Source: CAD feature listing. Evaluate the final solid. Frame: model axes, mm. A direction names the side the tool comes from. Give positions to 0.01 mm unless a question says otherwise; leave off trailing zeros. Put each result on its own line as item: value.
```python
from build123d import *
from build123d.topology import SkipClean

# Parameters (mm, degrees)
BOSS_EXTRUDE1_DEPTH = 640
SKETCH22_R          = 6
CUT_EXTRUDE4_DEPTH  = 10
BOSS_EXTRUDE2_DEPTH = 63
BOSS_EXTRUDE3_DEPTH = 7
SKETCH26_R          = 6
CUT_EXTRUDE5_DEPTH  = 7
FILLET1_R           = 10
FILLET2_R           = 10
FILLET3_R           = 5
FILLET5_R           = 1


with BuildPart() as part:
    # Sketch1 → Boss-Extrude1 (new body)
    with BuildSketch(Plane.XY):
        Polygon((0, 0), (0, 70), (70, 70), (70, 63), (7, 63), (7, 0), align=None)
    extrude(amount=BOSS_EXTRUDE1_DEPTH)

    # Sketch22 → Cut-Extrude4 (cut)
    with BuildSketch(Plane(origin=(0, 70, 0), x_dir=(1, 0, 0), z_dir=(0, 1, 0))):
        with Locations((35, 0)):
            Circle(SKETCH22_R)
        with Locations((35, 500)):
            Circle(SKETCH22_R)
        with Locations(Location((35, -500, 0), (0, 0, 270))):
            Circle(SKETCH22_R)
    extrude(amount=-CUT_EXTRUDE4_DEPTH, mode=Mode.SUBTRACT)

    # Sketch23 → Boss-Extrude2 (add)
    with BuildSketch(Plane(origin=(0, 0, 0), x_dir=(1, 0, 0), z_dir=(0, 1, 0))):
        Polygon((0, -640), (42.5, -713.612159322), (48.562177826, -710.112159322), (7, -640), align=None)
    extrude(amount=BOSS_EXTRUDE2_DEPTH)

    # Sketch25 → Boss-Extrude3 (add)
    with BuildSketch(Plane(origin=(0, 63, 0), x_dir=(1, 0, 0), z_dir=(0, 1, 0))):
        Polygon((70, -640), (0, -640), (42.5, -713.612159322), (70, -713.612159322), align=None)
    extrude(amount=BOSS_EXTRUDE3_DEPTH)

    # Sketch26 → Cut-Extrude5 (cut)
    with BuildSketch(Plane(origin=(-275.556719825, 0, 163.348804279), x_dir=(-0.5099316128113042, 0, -0.8602149442178172), z_dir=(0.8602149442178172, 0, -0.5099316128113042))):
        with Locations((-614.36248118, 31.5)):
            Circle(SKETCH26_R)
        with Locations((-575.367085589, 31.5)):
            Circle(SKETCH26_R)
    extrude(amount=-CUT_EXTRUDE5_DEPTH, mode=Mode.SUBTRACT)

    # Mirror1: part across plane


with BuildPart() as part_1:
    with SkipClean():  # the faces are left unmerged after this step: merging them gives an invalid solid
        add(part.part)
        add(part.part.mirror(Plane.XY))

    # Fillet1
    fillet1_edges = [part_1.edges().sort_by_distance(p)[0] for p in [
        (0, 35, 640),
        (0, 35, -640),
    ]]
    fillet(fillet1_edges, radius=FILLET1_R)

    # Fillet2
    fillet2_edges = [part_1.edges().sort_by_distance(p)[0] for p in [
        (7, 31.5, -640),
        (7, 31.5, 640),
    ]]
    fillet(fillet2_edges, radius=FILLET2_R)

    # Fillet3
    fillet3_edges = [part_1.edges().sort_by_distance(p)[0] for p in [
        (7, 63, 318.629374486),
        (7.355792038, 63, -639.902468471),
        (7.355792038, 63, 639.902468471),
        (28.480014192, 63, 676.235112211),
        (28.480014192, 63, -676.235112211),
    ]]
    fillet(fillet3_edges, radius=FILLET3_R)

    # Fillet5
    fillet5_edges = [part_1.edges().sort_by_distance(p)[0] for p in [
        (0, 70, 318.660254038),
        (0, 0, 318.660254038),
        (70, 70, 356.806079661),
        (21.919872981, 0, -677.966333699),
        (21.919872981, 0, 677.966333699),
        (0.340741737, 0, 639.908698527),
        (0.340741737, 0, -639.908698527),
        (21.919872981, 70, -677.966333699),
        (21.919872981, 70, 677.966333699),
        (0.340741737, 70, 639.908698527),
        (0.340741737, 70, -639.908698527),
        (7, 0, 318.629374486),
        (7.355792038, 0, 639.902468471),
        (7.355792038, 0, -639.902468471),
        (0, 70, 318.660254038),
        (0, 70, -318.660254038),
        (70, 70, 356.806079661),
        (70, 70, -356.806079661),
        (28.480014192, 0, 676.235112211),
        (28.480014192, 0, -676.235112211),
    ]]
    fillet(fillet5_edges, radius=FILLET5_R)


solid = part_1.part
```
(1) Line query: probe 1 along X at (y, z) = (65, -500); probe 2 along Y at (x, z) = (51, 227.5); probe 3 along X at (y, z) = (18, 595.5). Output: solid intervals per line, ascending. Write a range as from..to.
Calculated:
probe 1: x = 0..29, 41..70
probe 2: y = 63..70
probe 3: x = 0..7
(2) Reachability of faces 1 (the flat face through (28.76, 29.1, -676.71)), 2 (the flat face through (0, 35, 9)) from +Z, -Z, +X, -X, +Y, -Y: full face, straight path, thin tool, end or side. Return the list, or none.
Calculated:
face 1: +X, -Y
face 2: +Z, -Z, -X, +Y, -Y
(3) Draft query along Z for faces 3 (the flat face through (21.632, 34.524, -677.467)), 4 (the cylindrical face through (21.88, 0.3, 677.32)), 5 (the cylindrical face through (30.069, 61.574, -675.968)). Return one class per face: released by +Z, released by -Z, zero draft, split by the parting line, or undercut.
Calculated:
face 3: released by -Z
face 4: released by +Z
face 5: undercut
(4) First-contact query: P1, Ø6, axis at x = 47, y = 48, coming from the +Z side; P2, Ø1.5, axis at x = 8.5, z = -60.5, coming from the -Y side; P3, Ø5, axis at y = 37.5, z = 117.5, coming from the +X side; P4, Ø9.5, axis at x = 35, z = 500, coming from the -Y side. Flat tips, straight axial feed; report the tip coordinate or a pass-through.
Calculated:
P1: stops at z = 712.75
P2: stops at y = 60.63
P3: stops at x = 7
P4: passes through
